Autodesk Inventor part; units mm, degrees
ref_plane "YZ Plane" through (0, 0, 0) normal (1, 0, 0) x (0, 1, 0)
ref_plane "XZ Plane" through (0, 0, 0) normal (0, 1, 0) x (-1, 0, 0)
ref_plane "XY Plane" through (0, 0, 0) normal (0, 0, 1) x (1, 0, 0)
sketch "スケッチ1" plane through (0, 0, 0) normal (0, 1, 0) x (-1, 0, 0)
  line L0 (0, 0) -> (25, 0)
  line L1 (25, 0) -> (25, -33)
  line L2 (25, -33) -> (0, -33)
  line L3 (0, -33) -> (0, 0)
  line L4 (25, -27) -> (0, -33)
  dimension "d0" = 33
  dimension "d1" = 25
  dimension "d2" = 27
extrude "押し出し1" add sketch "スケッチ1" along normal blind 2.65
sketch "スケッチ2" plane through (0, 2.65, 0) normal (0, 1, 0) x (1, 0, 0)
  line L0 (0, 0) -> (0, 33)
  circle A0 centre (0, 33) radius 8
  dimension "d5" = 16
extrude "押し出し2" cut sketch "スケッチ2" against normal blind 2.65
sketch "スケッチ3" plane through (0, 2.65, 0) normal (0, 1, 0) x (1, 0, 0)
  line L0 (-25, 0) -> (0, 0)
  line L1 (-25, 0) -> (-12.3, 0)
  line L2 (-12.3, 0) -> (-12.3, -20)
  line L3 (-12.3, -20) -> (-25, -20)
  line L4 (-25, -20) -> (-25, 0)
  line L5 (0, 0) -> (0, 25)
  circle A0 centre (-12.3, 0) radius 2
  point P0 (-12.3, -2)
  point P1 (-14.3, 0)
  dimension "d8" = 20
  dimension "d9" = 12.3
  dimension "d10" = 4
extrude "押し出し3" add sketch "スケッチ3" against normal blind 2.65 contours A0 L2 L3 L4 L0
sketch "スケッチ4" plane through (0, 2.65, 0) normal (0, 1, 0) x (1, 0, 0)
  arc A0 (-14.3, 0) -> (-12.3, -2) centre (-12.3, 0) ccw
  line L0 (-12.3, -2) -> (-12.3, -20)
  circle A1 centre (-12.3, 0) radius 2
  point P0 (0, 0)
  point P1 (-14.3, 0)
extrude "押し出し4" cut sketch "スケッチ4" against normal blind 2.65
sketch "スケッチ5" plane through (0, 2.65, 0) normal (0, 1, 0) x (1, 0, 0)
  line L0 (-25, -20) -> (-12.3, -20)
  line L1 (-12.3, -20) -> (0, -20)
  line L2 (0, -20) -> (0, -12.5)
  line L3 (0, -12.5) -> (-12.3, -12.5)
  line L4 (-12.3, -12.5) -> (-12.3, -20)
  line L5 (-10.3, 0) -> (0, 0)
  dimension "d15" = 12.5
  dimension "d16" = 12.3
extrude "押し出し5" add sketch "スケッチ5" against normal blind 2.65
sketch "スケッチ6" plane through (0, 2.65, 0) normal (0, 1, 0) x (1, 0, 0)
  line L0 (-12.3, -12.5) -> (-12.3, -2)
  point P0 (0, 0)
hole "穴1" at (-12.3, 2.65, 12.5) direction (0, -1, 0) diameter 4 end through all
properties part number "bendpart_90deg"
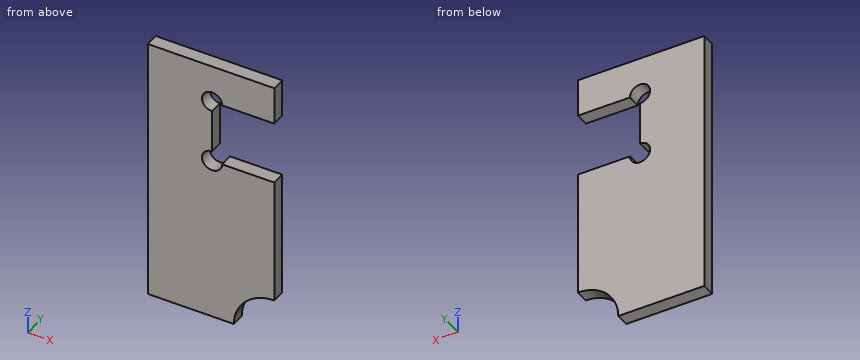
Source: CAD feature listing. Evaluate the final solid. Frame: model axes, mm. Give positions to 0.01 mm unless a question says otherwise; leave off trailing zeros. Order: outer loops, then holes, each group sorted by start corner. A loop starts at its lowest first (then second) coordinate and runs counter-clockwise, first axis right, second up. Notation, with made-up numbers: (32, -17) -> (81, -17) arc R27 ccw to (81, 16) -> close; hole circle Ø1 at (48.5, -38.75). An arc over 180 degrees is marked (long way). Use a Markdown table: item, result.
1) Ray query, line 1 along Z through (x, y) = (-10, 1.3); line 2 along Z through (x, y) = (-6, 1.15); line 3 along X through (y, z) = (0.9, -1). Return the intervals inside material, ascending. Write a range as [from, to].
Answer list:
| item | result |
|---|---|
| line 1 | [-33, 0], [12.5, 20] |
| line 2 | [-27.71, 0], [12.5, 20] |
| line 3 | [-25, -14.03], [-10.57, 0] |
2) Section query C-C, the plane y = 1. Return the cut outline in (x, z), then the cut area to 3 significant figures.
Answer list:
| item | result |
|---|---|
| outline | (-25, -33) -> (-8, -33) arc R8 cw to (0, -25) -> (0, 0) -> (-10.3, 0) arc R2 cw (long way) to (-12.3, 2) -> (-12.3, 10.5) arc R2 cw (long way) to (-10.3, 12.5) -> (0, 12.5) -> (0, 20) -> (-25, 20) -> close |
| area | 1,100 mm² |
3) Section query B-B, the plane z = 13. Return the cut outline in (x, y).
Answer list:
| item | result |
|---|---|
| outline | (-25, 0) -> (-14.24, 0) -> (-14.24, 2.65) -> (-25, 2.65) -> close; (-10.36, 0) -> (0, 0) -> (0, 2.65) -> (-10.36, 2.65) -> close |
4) Contact query for a flat-ended pin moving along its axis: P1, Ø1, axis at x = -5.5, y = 1.5, coming from the -Z side. Output: stop coordinate, or through.
Answer list:
| item | result |
|---|---|
| P1 | z = -27.71 |
5) Section query A-A, the plane x = -9.25. Return the cut outline in (y, z), then the cut area to 3 significant figures.
Answer list:
| item | result |
|---|---|
| outline | (0, -33) -> (2.65, -33) -> (2.65, 0) -> (0, 0) -> close; (0, 12.5) -> (2.65, 12.5) -> (2.65, 20) -> (0, 20) -> close |
| area | 107 mm² |
6) Section query D-D, the plane z = 4. Return the cut outline in (x, y).
Answer list:
| item | result |
|---|---|
| outline | (-25, 0) -> (-12.3, 0) -> (-12.3, 2.65) -> (-25, 2.65) -> close |
